```python
from build123d import *

# Parameters (mm, degrees)
SKETCH_1_R          = 4.1
EXTRUDE_1_DEPTH     = 65
SKETCH_2_R          = 4.923200542
EXTRUDE_2_DEPTH     = 3
SKETCH_3_R          = 1.25
CUT_EXTRUDE_1_DEPTH = 13
SKETCH_4_R          = 3.85
EXTRUDE_3_DEPTH     = 4
SKETCH_5_R          = 1.25
CUT_EXTRUDE_2_DEPTH = 14


with BuildPart() as part:
    # Эскиз1 → Бобышка-Вытянуть1 (new body)
    with BuildSketch(Plane.XY):
        with BuildLine():
            Line((5.123475383, -4), (32.5, -4))
            Line((32.5, -4), (32.5, 0))
            Line((32.5, 0), (6.5, 0))
            ThreePointArc((6.5, 0), (5.25594901, 3.824264635), (2, 6.184658438))
            Line((2, 6.184658438), (2, 19.184658438))
            Line((2, 19.184658438), (-2, 19.184658438))
            Line((-2, 19.184658438), (-2, 6.184658438))
            ThreePointArc((-2, 6.184658438), (-5.326428587, -3.725474266), (5.123475383, -4))
        make_face()
        Circle(SKETCH_1_R, mode=Mode.SUBTRACT)
    extrude(amount=EXTRUDE_1_DEPTH)

    # Эскиз2 → Бобышка-Вытянуть2 (add)
    with BuildSketch(Plane.XY.offset(65)):
        Circle(SKETCH_2_R)
    extrude(amount=-EXTRUDE_2_DEPTH)

    # Эскиз3 → Вырез-Вытянуть1 (cut)
    with BuildSketch(Plane(origin=(0, 0, 0), x_dir=(1, 0, 0), z_dir=(0, 1, 0))):
        with Locations((12.5, -5)):
            Circle(SKETCH_3_R)
        with Locations((28.5, -5)):
            Circle(SKETCH_3_R)
        with BuildLine():
            Line((27, -57.75), (30, -57.75))
            ThreePointArc((30, -57.75), (32.25, -60), (30, -62.25))
            Line((30, -62.25), (27, -62.25))
            ThreePointArc((27, -62.25), (24.75, -60), (27, -57.75))
        make_face()
        with BuildLine():
            Line((11, -57.75), (14, -57.75))
            ThreePointArc((14, -57.75), (16.25, -60), (14, -62.25))
            Line((14, -62.25), (11, -62.25))
            ThreePointArc((11, -62.25), (8.75, -60), (11, -57.75))
        make_face()
    extrude(amount=-CUT_EXTRUDE_1_DEPTH, mode=Mode.SUBTRACT)

    # Эскиз4 → Бобышка-Вытянуть3 (add)
    with BuildSketch(Plane.ZY.offset(2)):
        with Locations((8, 12.684658438)):
            Circle(SKETCH_4_R)
        with Locations((57, 12.684658438)):
            Circle(SKETCH_4_R)
    extrude(amount=EXTRUDE_3_DEPTH)

    # Эскиз5 → Вырез-Вытянуть2 (cut)
    with BuildSketch(Plane.ZY.offset(6)):
        with Locations((8, 12.684658438)):
            Circle(SKETCH_5_R)
        with Locations((56.916589889, 12.684658438)):
            Circle(SKETCH_5_R)
    extrude(amount=-CUT_EXTRUDE_2_DEPTH, mode=Mode.SUBTRACT)


solid = part.part
```
Geometry: final body of the model. Coordinates: model frame, mm. A direction names the side the tool comes from. Round coordinates to 2 decimals unless told otherwise and drop trailing zeros. Loops run counter-clockwise (first coordinate to the right, second up) from the corner with the lowest first, then second, coordinate; pieces in that order, holes last. Notation, with made-up numbers: (40, -36.5) -> (48, -36.5) arc R16 ccw to (48, -13.5) -> close; hole circle Ø11 at (35, 11.25). An arc over 180 degrees is marked (long way). Use one line per item in the form item = value. Start each with the question number.
1) Section D-D on y = 10.5. Output: boundary loops of the cut face in (x, z), then the cut area to 3 significant figures.
2) Draft query along X for faces 1 (the flat face through (29, -2, 62.25)), 2 (the flat face through (6, 2, 65)), 3 (the flat face through (-6, 14, 7)). Return one class per face: released by +X, released by -X, zero draft, split by the parting line, or undercut.
3) Section B-B on z = 46. Output: boundary loops of the cut face in (x, y), then the cut area to 3 significant figures.
4) Access query for faces 4 (the cylindrical face through (8.75, -1.97, 60.05)), 5 (the cylindrical face through (-0.534, 4.065, 30.566)), 6 (the flat face through (19, -4, 32)), 7 (the cylindrical face through (-3.972, 11.21, 60.556)). Directions: +Z, -Z, +X, -X, +Y, -Y. A direction counts if a zero-diameter tool reaches every point of the face in a straight line with its end or side. Return the directions, or none.
5) Section C-C on x = 28.5. Output: boundary loops of the cut face in (y, z), then the cut area to 3 significant figures.
6) Section A-A on z = 57. Output: boundary loops of the cut face in (x, y).
7) Line query: L1, parallel to Y at x = 0, z = 31; L2, parallel to Y at x = -3.5, z = 7; L3, parallel to X at y = -2.7, z = 5. Output: solid intervals per line, ascending.
8) First-contact query: P1, Ø4, axis at y = 12.68, z = 56.92, coming from the +X side; P2, Ø6.5, axis at x = 0.5, y = 0.5, coming from the -Z side; P3, Ø3, axis at x = 12.5, z = 5, coming from the -Y side. Flat tips, straight axial feed; report the tip coordinate or a pass-through.
Response:
q1.outline = (-6, 4.83) -> (-2, 4.83) -> (-2, 0) -> (2, 0) -> (2, 65) -> (-2, 65) -> (-2, 60.17) -> (-6, 60.17) -> (-6, 53.83) -> (-2, 53.83) -> (-2, 11.17) -> (-6, 11.17) -> close
q1.area = 311 mm^2
q2.face_1 = undercut
q2.face_2 = zero draft
q2.face_3 = released by -X
q3.outline = (-2, 6.18) arc R6.5 ccw (long way) to (5.12, -4) -> (32.5, -4) -> (32.5, 0) -> (6.5, 0) arc R6.5 ccw to (2, 6.18) -> (2, 19.18) -> (-2, 19.18) -> close; hole circle Ø8.2 at (0, 0)
q3.area = 237 mm^2
q4.face_4 = +Y, -Y
q4.face_5 = -Z
q4.face_6 = +Z, -Z, +X, -Y
q4.face_7 = -X
q5.outline = (-4, 0) -> (0, 0) -> (0, 3.75) -> (-4, 3.75) -> close; (-4, 6.25) -> (0, 6.25) -> (0, 57.75) -> (-4, 57.75) -> close; (-4, 62.25) -> (0, 62.25) -> (0, 65) -> (-4, 65) -> close
q5.area = 232 mm^2
q6.outline = (-6, 8.83) -> (-2, 8.83) -> (-2, 6.18) arc R6.5 ccw (long way) to (5.12, -4) -> (32.5, -4) -> (32.5, 0) -> (6.5, 0) arc R6.5 ccw to (2, 6.18) -> (2, 11.44) -> (-6, 11.44) -> close; (-6, 13.93) -> (2, 13.93) -> (2, 19.18) -> (-2, 19.18) -> (-2, 16.53) -> (-6, 16.53) -> close; hole circle Ø8.2 at (0, 0)
q7.L1 = -6.5 to -4.1, 4.1 to 19.18
q7.L2 = -5.48 to -2.14, 2.14 to 5.48, 8.97 to 11.93, 13.43 to 16.4
q7.L3 = -5.91 to -3.09, 3.09 to 11.25, 13.75 to 27.25, 29.75 to 32.5
q8.P1 = 2
q8.P2 = 62
q8.P3 = -4
